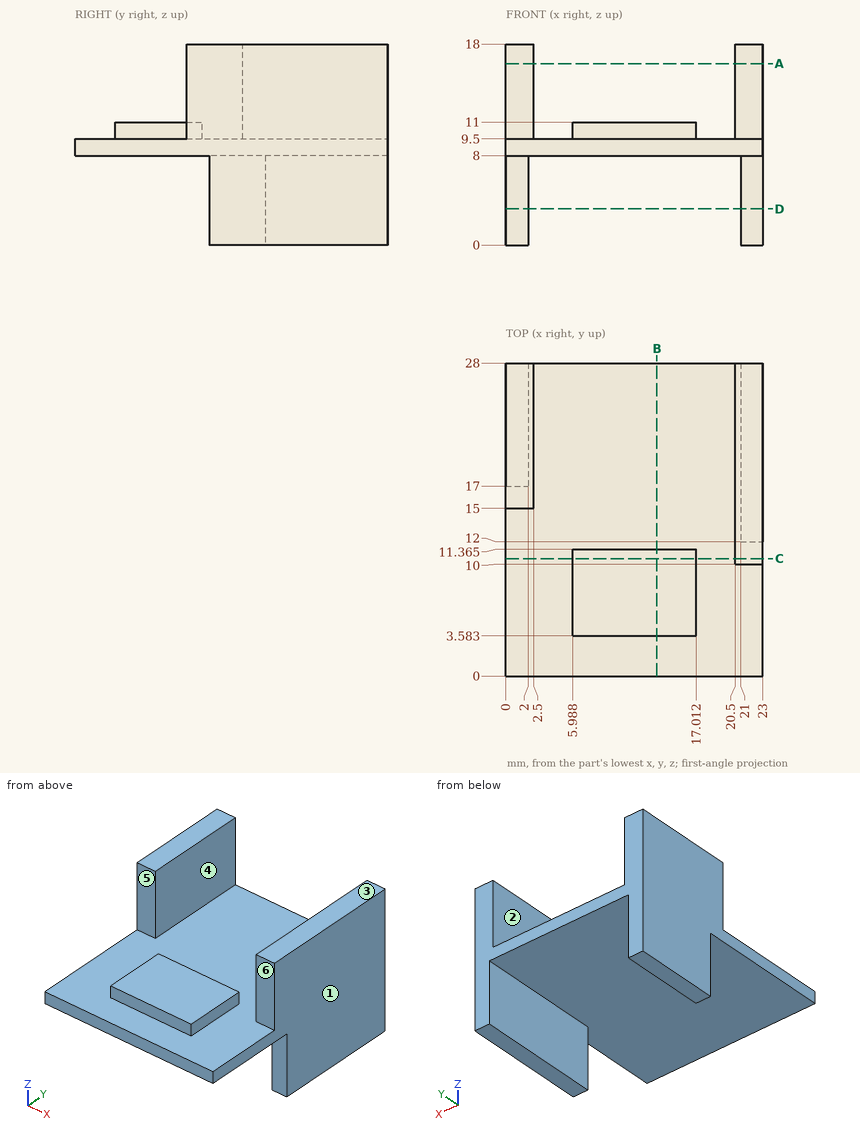
Could you check a few things on this drawing? It's one solid part, dimensions in mm from its lowest x, y, z. A direction names the side the tool comes from. Coordinates: 2 decimals unless noted, no trailing zeros. Write each loop counter-clockwise with the first axis right and the second up, starting at its lowest first coordinate (ties: lowest second). Pieces come first, ordered by that corner, then holes.
Q1. Imagine slicing it at C-C, the plane y = 10.5. List the corners of the cut face in (x, z) for me.
Results found:
outline: (0, 8) - (23, 8) - (23, 18) - (20.5, 18) - (20.5, 9.5) - (17.01, 9.5) - (17.01, 11) - (5.99, 11) - (5.99, 9.5) - (0, 9.5) - close
Q2. Which directions (+Z, -Z, +X, -X, +Y, -Y) give clear straight access to the entire face, cutting with the end or side of a thin tool? Please do the marked faces 4, 5 and 6.
Results found:
face 4: +Z, +Y, -Y
face 5: +Z, -X, -Y
face 6: +Z, +X, -Y
Q3. For P1, Ø2, axis at x = 18.5, y = 7.5, coming from the +Z side; P2, Ø5, axis at x = 6, y = 7.5, coming from the -Z side; P3, Ø1.2, axis at y = 7, z = 10.5, coming from the -X side, each with a flat end and sliding along its axis, tell me the tip position at first contact or that it passes through.
Results found:
P1: stops at z = 9.5
P2: stops at z = 8
P3: stops at x = 5.99
Q4. If we mould it in two halves opening along X, with no side actions, what happens to the marked faces 1, 2 and 3? For each: +X half, -X half, draft (parallel to the pull), parting line (faces both ways), or undercut.
Results found:
face 1: +X half
face 2: undercut
face 3: draft
Q5. Imagine slicing it at D-D, the plane z = 3.25. List the corners of the cut face in (x, y) for me.
Results found:
outline: (0, 17) - (2, 17) - (2, 28) - (0, 28) - close; (21, 12) - (23, 12) - (23, 28) - (21, 28) - close
Q6. Imagine slicing it at B-B, the plane x = 13.5. List the corners of the cut face in (y, z) for me (1 decimal).
Results found:
outline: (0, 8) - (28, 8) - (28, 9.5) - (11.4, 9.5) - (11.4, 11) - (3.6, 11) - (3.6, 9.5) - (0, 9.5) - close
Q7. Imagine slicing it at A-A, the plane z = 16.25. List the corners of the cut face in (x, y) for me, plus the area to 3 significant figures.
Results found:
outline: (0, 15) - (2.5, 15) - (2.5, 28) - (0, 28) - close; (20.5, 10) - (23, 10) - (23, 28) - (20.5, 28) - close
area: 77.5 mm2
Q8. Please list where these lines run through material, in increasing order: L1, parallel to X at y = 21.5, z = 11.5; L2, parallel to X at y = 26, z = 3.25; L3, parallel to Z at x = 17.25, y = 3.5.
Results found:
L1: x = 0 to 2.5, 20.5 to 23
L2: x = 0 to 2, 21 to 23
L3: z = 8 to 9.5
